Source: CAD feature listing. Evaluate the final solid. Frame: model axes, mm. A direction names the side the tool comes from. Round coordinates to 2 decimals unless told otherwise and drop trailing zeros. Write each loop counter-clockwise with the first axis right and the second up, starting at its lowest first coordinate (ties: lowest second). Pieces come first, ordered by that corner, then holes. Notation, with made-up numbers: (30.5, -29) -> (51.5, -29) arc R29 cw to (51.5, -7) -> close; hole circle Ø3 at (61.5, -14). An arc over 180 degrees is marked (long way). Put each result on its own line as item: value.
Autodesk Fusion 360 part; units mm, degrees
sketch "Sketch1" plane through (0, 0, 0) normal (0, 1, 0) x (1, 0, 0)
  line L0 (47, 36) -> (-47, 36)
  line L1 (-47, 36) -> (-47, -36)
  line L2 (-47, -36) -> (47, -36)
  line L3 (47, -36) -> (47, 36)
  line L4 (47, 36) -> (-47, -36) construction
  line L5 (-47, 36) -> (47, -36) construction
  dimension "d1" = 72
  dimension "d2" = 94
extrude "Extrude1" add sketch "Sketch1" along normal blind 5
sketch "Sketch2" plane through (0, 5, 0) normal (0, 1, 0) x (-1, 0, 0)
  line L0 (-47, 36) -> (-47, -36)
  line L1 (-47, -36) -> (47, -36)
  line L2 (47, -36) -> (47, 36)
  line L3 (47, 36) -> (-47, 36)
  line L4 (-41.6, -30.6) -> (41.6, -30.6)
  line L5 (41.6, -30.6) -> (41.6, 30.6)
  line L6 (41.6, 30.6) -> (-41.6, 30.6)
  line L7 (-41.6, 30.6) -> (-41.6, -30.6)
  line L8 (-41.6, -30.6) -> (41.6, 30.6) construction
  line L9 (41.6, -30.6) -> (-41.6, 30.6) construction
  dimension "d5" = 83.2
  dimension "d6" = 61.2
extrude "Extrude2" add sketch "Sketch2" along normal blind 9.8 contours L4 L5 L6 L7
fillet "Fillet1" radius 2 4 edges at (47, 2.5, -36) (47, 2.5, 36) (-47, 2.5, 36) (-47, 2.5, -36)
fillet "Fillet2" radius 2 8 edges at (0, 0, -36) (-46.4142, 0, -35.4142) (-47, 0, 0) (-46.4142, 0, 35.4142) (0, 0, 36) (46.4142, 0, 35.4142) (47, 0, 0) (46.4142, 0, -35.4142)
sketch "Sketch3" plane through (0, 14.8, 0) normal (0, 1, 0) x (-1, 0, 0)
  line L0 (-41.6, 30.6) -> (-41.6, -30.6)
  line L1 (-41.6, -30.6) -> (41.6, -30.6)
  line L2 (41.6, -30.6) -> (41.6, 30.6)
  line L3 (41.6, 30.6) -> (-41.6, 30.6)
  line L4 (-38.6, -28) -> (38.6, -28)
  line L5 (38.6, -28) -> (38.6, 28)
  line L6 (38.6, 28) -> (-38.6, 28)
  line L7 (-38.6, 28) -> (-38.6, -28)
  line L8 (-38.6, -28) -> (38.6, 28) construction
  line L9 (38.6, -28) -> (-38.6, 28) construction
  line L10 (-45, -34) -> (45, -34)
  dimension "d11" = 56
  dimension "d12" = 77.2
  dimension "d13" = 90
extrude "Extrude3" cut sketch "Sketch3" against normal blind 9.8 contours L4 L5 L6 L7
sketch "Sketch4" plane through (0, 0, -30.6) normal (0, 0, -1) x (-1, 0, 0)
  line L0 (-41.6, 5) -> (41.6, 5)
  line L1 (41.6, 5) -> (41.6, 14.8)
  line L2 (41.6, 14.8) -> (-41.6, 14.8)
  line L3 (-41.6, 14.8) -> (-41.6, 5)
  line L4 (10, 14) -> (-10, 14)
  line L5 (-10, 14) -> (-10, 12)
  line L6 (-10, 12) -> (10, 12)
  line L7 (10, 12) -> (10, 14)
  line L8 (10, 14) -> (-10, 12) construction
  line L9 (-10, 14) -> (10, 12) construction
  point P0 (0, 13)
  dimension "d16" = 20
  dimension "d17" = 2
extrude "Extrude4" add sketch "Sketch4" along normal blind 1.2 contours L4 L5 L6 L7
sketch "Sketch5" plane through (10, 0, 0) normal (1, 0, 0) x (0, 0, -1)
  line L0 (30.6, 14) -> (30.6, 12)
  line L1 (30.6, 12) -> (31.8, 12)
  line L2 (31.8, 12) -> (31.8, 14)
  line L3 (31.8, 14) -> (30.6, 14)
  point P0 (31.8, 14)
  point P1 (31.8, 12)
  point P2 (31.8, 12)
  point P3 (31.8, 12)
  point P4 (31.8, 12)
  point P5 (31.8, 12)
  point P6 (31.8, 14)
  point P7 (31.8, 14)
  point P8 (31.8, 14)
  point P9 (31.8, 14)
  point P10 (31.8, 14)
  point P11 (31.8, 14)
  point P12 (31.8, 14)
  point P13 (31.8, 14)
  point P14 (31.8, 14)
  point P15 (31.8, 14)
  point P16 (31.8, 12)
  point P17 (31.8, 14)
  point P18 (31.8, 12)
  point P19 (31.8, 14)
ref_plane "WorkPlane2" through (0, 9.9, 0) normal (0, 0, 1) x (-1, 0, 0)
ref_plane "WorkPlane1" through (0, 9.9, 30.6) normal (0, 0, 1) x (1, 0, 0)
ref_plane "WorkPlane3" through (0, 13, -26.8) normal (0, 0, -1) x (-1, 0, 0)
ref_plane "WorkPlane4" through (0, 13, -26.8) normal (0, 0, -1) x (-1, 0, 0)
mirror "Mirror1" about plane through (0, 9.9, 0) normal (0, 0, 1) of "Extrude4"
chamfer "Chamfer1" distance 1 angle 45 2 edges at (0, 14, 31.8) (0, 12, 31.8)
chamfer "Chamfer2" distance 1 angle 45 2 edges at (0, 14, -31.8) (0, 12, -31.8)
sketch "Sketch6" plane through (0, 14.8, 0) normal (0, 1, 0) x (-1, 0, 0)
  line L0 (38.6, -28) -> (-38.6, -28)
  line L1 (-38.6, -28) -> (-38.6, 28)
  line L2 (-38.6, 28) -> (38.6, 28)
  line L3 (38.6, 28) -> (38.6, -28)
  line L4 (-41.6, 30.6) -> (-41.6, -30.6)
  line L5 (-41.6, -30.6) -> (41.6, -30.6)
  line L6 (41.6, -30.6) -> (41.6, 30.6)
  line L7 (41.6, 30.6) -> (-41.6, 30.6)
  point P0 (42.1144, 28)
  point P1 (-41.6, 30.6)
Q1. Cut plane C-C on y = 9.25. Output: boundary loops of the cut face in (x, z).
Ans:
outline: (-41.6, -30.6) -> (41.6, -30.6) -> (41.6, 30.6) -> (-41.6, 30.6) -> close; hole (-38.6, -28) -> (38.6, -28) -> (38.6, 28) -> (-38.6, 28) -> close
Q2. Draft query along Z for faces 1 (the flat face through (47, 3, 0)), 2 (the flat face through (1, 10, -28)), 3 (the cylindrical face through (46.43, 3.52, -35.4)). Return one class per face: +Z half, -Z half, draft (parallel to the pull), parting line (faces both ways), or undercut.
Ans:
face 1: draft
face 2: undercut
face 3: -Z half
Q3. Material intervals for line 1 (Z direction, x = -21, y = 7); line 2 (X direction, y = 7.5, z = 7); line 3 (Y direction, x = -35, z = 14), sorted ascending. Write a range as [from, to].
Ans:
line 1: z = [-30.6, -28], [28, 30.6]
line 2: x = [-41.6, -38.6], [38.6, 41.6]
line 3: y = [0, 5]
Q4. Reachability of faces 4 (the flat face through (1, 5, 0)), 5 (the flat face through (-41.6, 10, 0)), 6 (the flat face through (41.6, 10, 0)), 7 (the flat face through (1, 3, -36)) from +Z, -Z, +X, -X, +Y, -Y: full face, straight path, thin tool, end or side. Return the list, or none.
Ans:
face 4: +Y
face 5: +Z, -Z, -X, +Y
face 6: +Z, -Z, +X, +Y
face 7: -Z, +X, -X, +Y, -Y
Q5. Cut plane B-B on z = -1. Output: boundary loops of the cut face in (x, y).
Ans:
outline: (-47, 2) arc R2 ccw to (-45, 0) -> (45, 0) arc R2 ccw to (47, 2) -> (47, 5) -> (41.6, 5) -> (41.6, 14.8) -> (38.6, 14.8) -> (38.6, 5) -> (-38.6, 5) -> (-38.6, 14.8) -> (-41.6, 14.8) -> (-41.6, 5) -> (-47, 5) -> close
Q6. Pin query (flat end, axial travel): pin 1 (1 mm diameter, centred on y = 13.5, z = -31, fed in from +X); pin 2 (1.3 mm diameter, centred on y = 13, z = -31, fed in from -X); pin 3 (6 mm diameter, centred on x = 18.5, y = 11.5, fed in from +Z). Return the tip coordinate at first contact, or that it passes through.
Ans:
pin 1: stops at x = 41.6
pin 2: stops at x = -41.6
pin 3: stops at z = 30.6
Q7. Cut plane A-A on x = -19.5. Output: boundary loops of the cut face in (y, z), and give its area (3 significant figures).
Ans:
outline: (0, -34) arc R2 ccw to (2, -36) -> (5, -36) -> (5, -30.6) -> (14.8, -30.6) -> (14.8, -28) -> (5, -28) -> (5, 28) -> (14.8, 28) -> (14.8, 30.6) -> (5, 30.6) -> (5, 36) -> (2, 36) arc R2 ccw to (0, 34) -> close
area: 409 mm^2
